Build history of the part. All positions in model axes, mm. Face numbers are marked on the shaded views. A direction names the side the tool comes from. Coordinates: 2 decimals unless noted, no trailing zeros. Write each loop counter-clockwise with the first axis right and the second up, starting at its lowest first coordinate (ties: lowest second). Pieces come first, ordered by that corner, then holes.
```python
from build123d import *

# Parameters (mm, degrees)
F0_W      = 104.1721515357
F0_H      = 71.7630404979
F1_DEPTH  = 254
F1_FACE_W = 254
F1_FACE_H = 71.7630404979
F2_R      = 25.449665143
F2_R_2    = 11.4170803912
F3_DEPTH  = 25.4
F4_W      = 21.7701625079
F4_H      = 73.5019464046
F4_H_2    = 26.9834827632
F5_DEPTH  = 25.4


with BuildPart() as f1:
    # F0 (on Front) → F1 (new body)
    with BuildSketch(Plane.XZ):
        with Locations((7.3065180331, 8.8980374858)):
            Rectangle(F0_W, F0_H)
    extrude(amount=F1_DEPTH)

    # F1_face (on face) + F2 (on Right) → F3 (join)
    with BuildSketch(Plane(origin=(-44.7795577347, -127, 8.8980374858), x_dir=(0, -1, 0), z_dir=(-1, 0, 0))):
        Rectangle(F1_FACE_W, F1_FACE_H)
    with BuildSketch(Plane.YZ):
        with Locations((-35.3816822171, -13.4047763422)):
            Circle(F2_R)
        with Locations((-35.3816822171, -13.4047763422)):
            Circle(F2_R_2, mode=Mode.SUBTRACT)
    extrude(amount=F3_DEPTH, dir=(-1, 0, 0))

    # F4 (on face) → F5 (join)
    with BuildSketch(Plane(origin=(-70.1795577347, 0, 0), x_dir=(0, -1, 0), z_dir=(-1, 0, 0))):
        with Locations((36.9942905381, -63.7344559655)):
            Rectangle(F4_W, F4_H)
        with Locations((36.9942905381, -13.4917413816)):
            Rectangle(F4_W, F4_H_2)
    extrude(amount=F5_DEPTH)


solid = f1.part
```
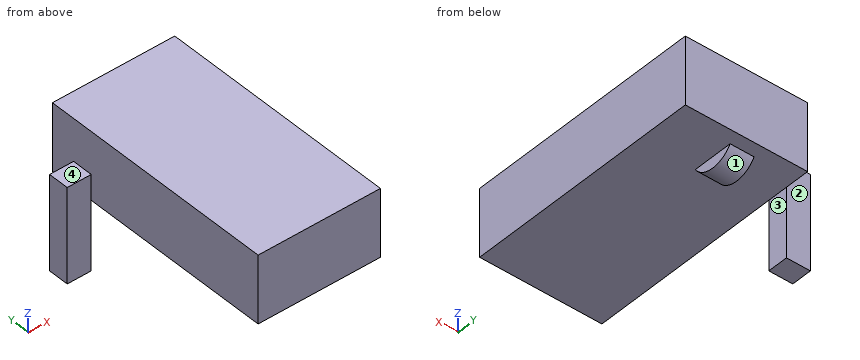
1. Saw through at B-B on y = -20. List the corners of the cut face in (x, z), plus the area to 3 significant figures.
Computed values:
outline: (-70.18, -26.98) - (-25.4, -26.98) - (-25.4, -33.68) - (0, -33.68) - (0, -26.98) - (59.39, -26.98) - (59.39, 44.78) - (-70.18, 44.78) - close
area: 9,470 mm2
2. Flat gauge pins, fed straight in: pin 1 (12.5 mm diameter, centred on x = -79, z = -25.5, fed in from +Y); pin 2 (6.5 mm diameter, centred on x = -82.5, y = -33.5, fed in from +Z); pin 3 (21.5 mm diameter, centred on y = -151.5, z = 6.5, fed in from -X); pin 4 (8 mm diameter, centred on x = -46.5, z = 6.5, fed in from +Y). Where does each tip first touch, or does it go through?
Computed values:
pin 1: stops at y = -26.11
pin 2: stops at z = 0
pin 3: stops at x = -70.18
pin 4: stops at y = 0
3. Saw through at C-C on z = -57. List the corners of the cut face in (x, y).
Computed values:
outline: (-95.58, -47.88) - (-70.18, -47.88) - (-70.18, -26.11) - (-95.58, -26.11) - close
4. Probe line 1 along Z through (x, y) = (13.5, -202); line 2 along X through (y, z) = (-168, 9); line 3 along Z through (x, y) = (-88, -38). List the from-to ranges inside material, lowest first.
Computed values:
line 1: z = -26.98 to 44.78
line 2: x = -70.18 to 59.39
line 3: z = -100.49 to 0
5. Saw through at D-D on x = -81. List the corners of the cut face in (y, z), plus the area to 3 significant figures.
Computed values:
outline: (-47.88, -100.49) - (-26.11, -100.49) - (-26.11, 0) - (-47.88, 0) - close
area: 2,190 mm2
6. Saw through at A-A on x = -12. List the corners of the cut face in (y, z).
Computed values:
outline: (-254, -26.98) - (-56.91, -26.98) arc R25.45 ccw to (-13.86, -26.98) - (0, -26.98) - (0, 44.78) - (-254, 44.78) - close
7. 3-axis set-ups, long thin cutter, end or side, ignore diameter. For the marked faces 1, 2, 3 and 4: which of +Z, -Z, +X, -X, +Y, -Y reach the whole face in a straight line?
Computed values:
face 1: -Z, +X
face 2: +Z, -Z, -X, +Y
face 3: -Z, +Y, -Y
face 4: +Z, -X, +Y, -Y
